Part model, mm, in its own coordinate system. A direction names the side the tool comes from. Round coordinates to 2 decimals unless told otherwise and drop trailing zeros. Loops run counter-clockwise (first coordinate to the right, second up) from the corner with the lowest first, then second, coordinate; pieces in that order, holes last. Notation, with made-up numbers: M 3.25,49 L 23.25,49 A22 ccw 23.25,73 Z; hole C 38,40.5 d3. An arc over 180 degrees is marked long. Write each question's results on one line, items separated by ' | '.
from build123d import *

# Parameters (mm, degrees)
SKETCH_1_R      = 6
SKETCH_1_R_2    = 5.25
EXTRUDE_2_DEPTH = 30
SKETCH_2_R      = 7.5
EXTRUDE_3_DEPTH = 3
SKETCH_3_R      = 5
EXTRUDE_4_DEPTH = 120
EXTRUDE_6_DEPTH = 4


with BuildPart() as part:
    # 草图1 → 凸台-拉伸2 (new body)
    with BuildSketch(Plane(origin=(0, 0, 0), x_dir=(1, 0, 0), z_dir=(0, 1, 0))):
        with Locations(Location((0, 0, 0), (0, 0, 270))):
            Circle(SKETCH_1_R)
        with Locations(Location((0, 0, 0), (0, 0, 270))):
            Circle(SKETCH_1_R_2, mode=Mode.SUBTRACT)
    extrude(amount=EXTRUDE_2_DEPTH)

    # 草图2 → 凸台-拉伸3 (add)
    with BuildSketch(Plane(origin=(0, 30, 0), x_dir=(1, 0, 0), z_dir=(0, 1, 0))):
        with Locations(Location((0, 0, 0), (0, 0, 270))):
            Circle(SKETCH_2_R)
    extrude(amount=EXTRUDE_3_DEPTH)

    # 草图3 → 凸台-拉伸4 (add)
    with BuildSketch(Plane(origin=(0, 33, 0), x_dir=(1, 0, 0), z_dir=(0, 1, 0))):
        with Locations(Location((0, 0, 0), (0, 0, 270))):
            Circle(SKETCH_3_R)
    extrude(amount=EXTRUDE_4_DEPTH)

    # 草图4 → 凸台-拉伸6 (add)
    with BuildSketch(Plane(origin=(0, 33, 0), x_dir=(1, 0, 0), z_dir=(0, 1, 0))):
        with BuildLine():
            Line((6, 1), (4.898979486, 1))
            ThreePointArc((4.898979486, 1), (4.974680765, 0.50254481), (5, 0))
            Line((5, 0), (6, 0))
            Line((6, 0), (6, 1))
        make_face()
        with BuildLine():
            ThreePointArc((5, 0), (4.974680765, -0.50254481), (4.898979486, -1))
            Line((4.898979486, -1), (6, -1))
            Line((6, -1), (6, 0))
            Line((6, 0), (5, 0))
        make_face()
    extrude(amount=EXTRUDE_6_DEPTH)


solid = part.part
Item 1: Which spindle directions (+Z, -Z, +X, -X, +Y, -Y) get a long thin tool onto all of the face, cutting with end or side? Do faces 4 (the flat face through (-4, 0, 4)), 5 (the cylindrical face through (-4.88, 92.16, -1.08)), 6 (the flat face through (0, 30, 0)). Say none if no direction does.
Filled sheet:
face 4: +Z, -Z, +X, -X, -Y | face 5: +Y | face 6: -Y
Item 2: Band-saw the part on D-D on y = 35. Give the cut face in (x, z).
Filled sheet:
outline: M 4.9,-1 L 6,-1 L 6,1 L 4.9,1 A5 ccw long Z
Item 3: Drop flat-ended pins along their axis: P1, Ø8, axis at y = 44.5, z = 5.5, coming from the -X side; P2, Ø6, axis at y = 52, z = 4, coming from the +X side; P3, Ø0.9, axis at x = 5.5, z = -0.5, coming from the +Y side; P4, Ø4, axis at x = 4, z = -0.5, coming from the -Y side. Give the stop position or say it passes through.
Filled sheet:
P1: x = -4.77 | P2: x = 4.9 | P3: y = 37 | P4: y = 0
Item 4: Band-saw the part on A-A on y = 59. Give the cut face in (x, z), and give its area (3 significant figures).
Filled sheet:
outline: C 0,0 d10 | area: 78.5 mm^2
Item 5: Band-saw the part on C-C on z = -3.5. Give the cut face in (x, y), and give its area (3 significant figures).
Filled sheet:
outline: M -6.63,30 L -4.87,30 L -4.87,0 L -3.91,0 L -3.91,30 L 3.91,30 L 3.91,0 L 4.87,0 L 4.87,30 L 6.63,30 L 6.63,33 L 3.57,33 L 3.57,153 L -3.57,153 L -3.57,33 L -6.63,33 Z | area: 954 mm^2
Item 6: Band-saw the part on B-B on x = -1.25. Give the cut face in (y, z), and give its area (3 significant figures).
Filled sheet:
outline: M 0,-5.87 L 30,-5.87 L 30,-7.4 L 33,-7.4 L 33,-4.84 L 153,-4.84 L 153,4.84 L 33,4.84 L 33,7.4 L 30,7.4 L 30,5.87 L 0,5.87 L 0,5.1 L 30,5.1 L 30,-5.1 L 0,-5.1 Z | area: 1,250 mm^2
Item 7: Two-plate mould, pull along Z, no slides. Class faces 1 (the cylindrical face through (1.6, 14.8, 5)), 2 (the cylindrical face through (1.802, 14.79, 5.723)), 3 (the flat face through (6, 30, 2)): +Z half, -Z half, draft (parallel to the pull), parting line (faces both ways), or undercut.
Filled sheet:
face 1: undercut | face 2: parting line | face 3: draft
Item 8: Wall check: L1, parallel to X at y = 9.5, z = 0; L2, parallel to Y at x = -5, z = -5; L3, parallel to Y at x = -2, z = -0.5. Give the ranges that are in metal, low to high.
Filled sheet:
L1: -6 to -5.25, 5.25 to 6 | L2: 30 to 33 | L3: 30 to 153
